The model under review builds one solid part; all positions refer to its coordinate system, in mm. A direction names the side the tool comes from. Give positions to 0.01 mm unless a question says otherwise; leave off trailing zeros. Order: outer loops, then holes, each group sorted by start corner. A loop starts at its lowest first (then second) coordinate and runs counter-clockwise, first axis right, second up.
```python
from build123d import *

# Parameters (mm, degrees)
SKETCH1_W               = 120
SKETCH1_H               = 100
BOSS_EXTRUDE1_DEPTH     = 40
SHELL1_T                = -5
SKETCH2_R               = 1.5
CUT_EXTRUDE1_DEPTH      = 86.586213843
SKETCH4_R               = 1.5
BOSS_EXTRUDE2_DEPTH     = 3
SKETCH7_R               = 5
CUT_EXTRUDE2_DEPTH      = 5
SKETCH8_R               = 1.475
CUT_EXTRUDE3_DEPTH      = 10
MIRROR2_COPY_1_SKETCH_R = 1.475
MIRROR2_COPY_1_DEPTH    = 10
FILLET1_R               = 2


with BuildPart() as part:
    # Sketch1 → Boss-Extrude1 (new body)
    with BuildSketch(Plane(origin=(0, 0, 0), x_dir=(1, 0, 0), z_dir=(0, 1, 0))):
        Rectangle(SKETCH1_W, SKETCH1_H)
    extrude(amount=BOSS_EXTRUDE1_DEPTH)

    # Shell1
    shell1_openings = [part.faces().sort_by_distance(p)[0] for p in [
        (0, 40, 0),
    ]]
    offset(amount=SHELL1_T, openings=shell1_openings, kind=Kind.INTERSECTION)

    # Sketch2 → Cut-Extrude1 (cut, through all)
    with BuildSketch(Plane(origin=(0, 5, 0), x_dir=(1, 0, 0), z_dir=(0, 1, 0))):
        with Locations(Location((-45, 35, 0), (0, 0, 270))):
            Circle(SKETCH2_R)
        with Locations(Location((45, 35, 0), (0, 0, 90))):
            Circle(SKETCH2_R)
        with Locations(Location((45, -35, 0), (0, 0, 270))):
            Circle(SKETCH2_R)
        with Locations(Location((-45, -35, 0), (0, 0, 90))):
            Circle(SKETCH2_R)
    extrude(amount=-CUT_EXTRUDE1_DEPTH, mode=Mode.SUBTRACT)

    # Sketch4 → Boss-Extrude2 (add)
    # profile 1 of 2: a face of its own
    with BuildSketch(Plane.XZ):
        with BuildLine():
            Line((60, 6), (67, 6))
            ThreePointArc((67, 6), (73, 0), (67, -6))
            Line((67, -6), (60, -6))
            Line((60, -6), (60, 6))
        make_face()
        with Locations(Location((67, 0, 0), (0, 0, 270))):
            Circle(SKETCH4_R, mode=Mode.SUBTRACT)
    # profile 2 of 2: a face of its own
    with BuildSketch(Plane.XZ):
        with BuildLine():
            Line((-60, 6), (-60, -6))
            Line((-60, -6), (-67, -6))
            ThreePointArc((-67, -6), (-73, 0), (-67, 6))
            Line((-67, 6), (-60, 6))
        make_face()
        with Locations(Location((-67, 0, 0), (0, 0, 90))):
            Circle(SKETCH4_R, mode=Mode.SUBTRACT)
    extrude(amount=-BOSS_EXTRUDE2_DEPTH)

    # Sketch7 → Cut-Extrude2 (cut)
    with BuildSketch(Plane.ZY.offset(60)):
        with Locations((-39.349087079, 10.249467904)):
            Circle(SKETCH7_R)
    extrude(amount=-CUT_EXTRUDE2_DEPTH, mode=Mode.SUBTRACT)

    # Sketch8 → Cut-Extrude3 (cut)
    with BuildSketch(Plane(origin=(0, 40, 0), x_dir=(1, 0, 0), z_dir=(0, 1, 0))):
        with Locations(Location((-57.5, 47.5, 0), (0, 0, 270))):
            Circle(SKETCH8_R)
    cut_extrude3 = extrude(amount=-CUT_EXTRUDE3_DEPTH, mode=Mode.SUBTRACT)

    # Mirror1: Cut-Extrude3 across plane
    add(cut_extrude3.mirror(Plane(origin=(0, 0, 0), x_dir=(0, 0, 1), z_dir=(1, 0, 0))), mode=Mode.SUBTRACT)

    # Mirror2: Cut-Extrude3 across plane
    add(cut_extrude3.mirror(Plane.XY), mode=Mode.SUBTRACT)

    # Mirror2 copy 1 sketch → Mirror2 copy 1 (cut)
    with BuildSketch(Plane(origin=(0, 40, 0), x_dir=(-1, 0, 0), z_dir=(0, 1, 0))):
        with Locations(Location((-57.5, 47.5, 0), (0, 0, 270))):
            Circle(MIRROR2_COPY_1_SKETCH_R)
    extrude(amount=-MIRROR2_COPY_1_DEPTH, mode=Mode.SUBTRACT)

    # Fillet1
    fillet1_edges = [part.edges().sort_by_distance(p)[0] for p in [
        (60, 20, 50),
        (-60, 20, 50),
        (-60, 20, -50),
        (60, 20, -50),
    ]]
    fillet(fillet1_edges, radius=FILLET1_R)


solid = part.part
```
Item 1: Draft analysis for pull direction X (two halves, no side actions). For faces 1 (the cylindrical face through (56.256, 35.07, 46.707)), 2 (the flat face through (65, 3, 0)), 3 (the cylindrical face through (-73, 1, 0)), 4 (the cylindrical face through (56.256, 35.07, -46.707)), state which applies: released by +X, released by -X, zero draft, split by the parting line, or undercut.
Values found:
face 1: undercut
face 2: zero draft
face 3: released by -X
face 4: undercut
Item 2: Clearance check with flat-ended pins moving along their axes: pin 1 Ø1 at (x, z) = (49.5, 37.5) entering from +Y; pin 2 Ø2.5 at (x, z) = (-58, 47.5) entering from +Y; pin 3 Ø2.5 at (x, z) = (57.5, 47.5) entering from +Y; pin 4 Ø6 at (x, z) = (64.5, -0.5) entering from +Y. State where each tip first meets the part, or that it passes through.
Values found:
pin 1: stops at y = 5
pin 2: stops at y = 40
pin 3: stops at y = 30
pin 4: stops at y = 3
Item 3: Take a section at A-A (x = 45). Give the boundary of the cut face in (y, z), and give its area (3 significant figures).
Values found:
outline: (0, -50) - (40, -50) - (40, -45) - (5, -45) - (5, -36.5) - (0, -36.5) - close; (0, -33.5) - (5, -33.5) - (5, 33.5) - (0, 33.5) - close; (0, 36.5) - (5, 36.5) - (5, 45) - (40, 45) - (40, 50) - (0, 50) - close
area: 820 mm2
Item 4: Take a section at C-C (z = 35). Give the boundary of the cut face in (x, y).
Values found:
outline: (-60, 0) - (-46.5, 0) - (-46.5, 5) - (-55, 5) - (-55, 40) - (-60, 40) - close; (-43.5, 0) - (43.5, 0) - (43.5, 5) - (-43.5, 5) - close; (46.5, 0) - (60, 0) - (60, 40) - (55, 40) - (55, 5) - (46.5, 5) - close
Item 5: For line 1 (X direction, y = 35, z = 47.5) (3 decimals); line 2 (X direction, y = 1.4, z = 0); line 3 (X direction, y = 12, z = 9.5), list the stretches that pass through material, from the lowest coordinate up.
Values found:
line 1: x = -60 to -58.975, -56.025 to 56.025, 58.975 to 60
line 2: x = -73 to -68.5, -65.5 to 65.5, 68.5 to 73
line 3: x = -60 to -55, 55 to 60
Item 6: Take a section at B-B (y = 24). Give the boundary of the cut face in (x, z), and give its area (3 significant figures).
Values found:
outline: (-60, -48) arc R2 ccw to (-58, -50) - (58, -50) arc R2 ccw to (60, -48) - (60, 48) arc R2 ccw to (58, 50) - (-58, 50) arc R2 ccw to (-60, 48) - close; hole (-55, -45) - (55, -45) - (55, 45) - (-55, 45) - close
area: 2,100 mm2
Item 7: For faces 5 (the flat face through (64, 1, -6)), 6 (the flat face through (-64, 1, 6)), 7 (the flat face through (57, 30, 48)), list the 3-axis set-ups (+Z, -Z, +X, -X, +Y, -Y) from which the entire face can be reached by the end or side of a thin tool; tool diameter is ignored.
Values found:
face 5: -Z, +X, +Y, -Y
face 6: +Z, -X, +Y, -Y
face 7: +Y
Item 8: Take a section at D-D (y = 35). Give the boundary of the cut face in (x, z) (3 decimals), and give its area (3 significant figures).
Values found:
outline: (-60, -48) arc R2 ccw to (-58, -50) - (58, -50) arc R2 ccw to (60, -48) - (60, 48) arc R2 ccw to (58, 50) - (-58, 50) arc R2 ccw to (-60, 48) - close; hole circle Ø2.95 at (-57.5, -47.5); hole circle Ø2.95 at (-57.5, 47.5); hole (-55, -45) - (55, -45) - (55, 45) - (-55, 45) - close; hole circle Ø2.95 at (57.5, -47.5); hole circle Ø2.95 at (57.5, 47.5)
area: 2,070 mm2
